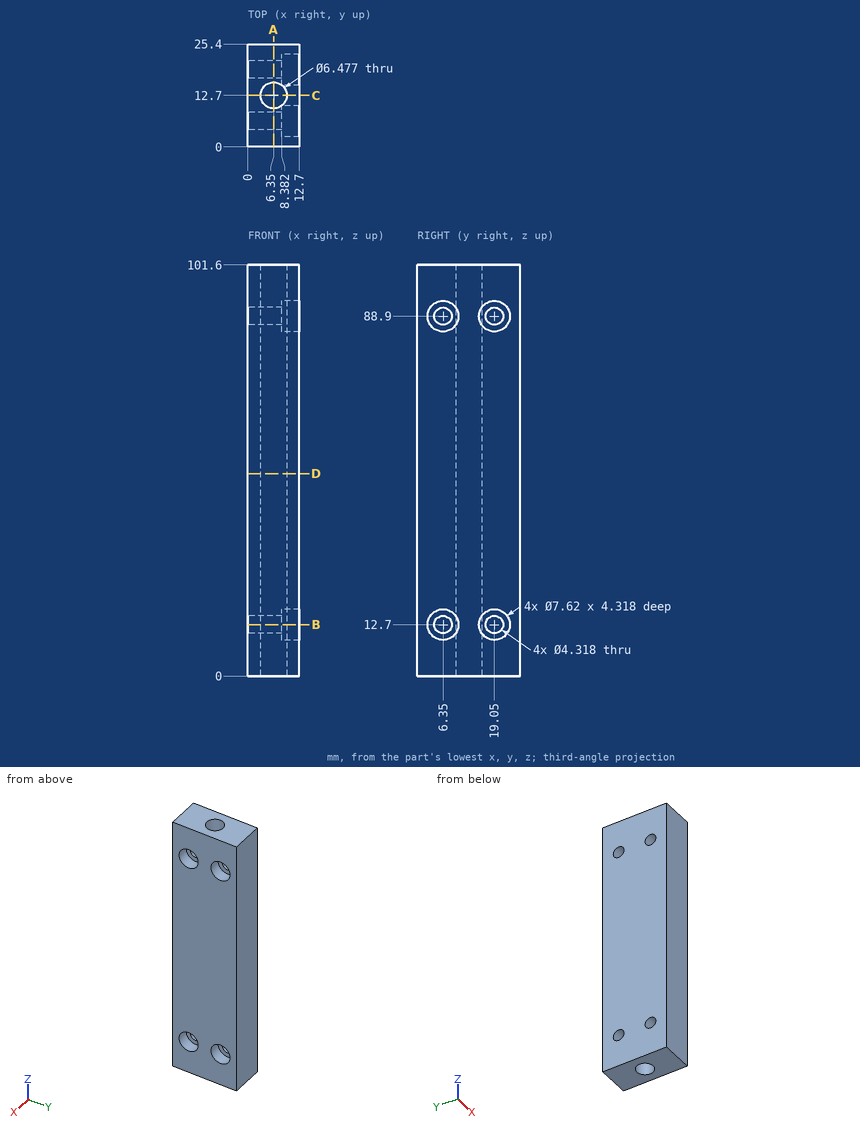
Part print with two shaded views. Sizes in mm from the minimum x, y, z corner. Coordinates: 2 decimals unless noted, no trailing zeros. Order: outer loops, then holes, each group sorted by start corner. A loop starts at its lowest first (then second) coordinate and runs counter-clockwise, first axis right, second up. Notation, with made-up numbers: M 5.5,55 L 38.5,55 A29 ccw 38.5,80 Z; hole C 55.25,20 d3. An arc over 180 degrees is marked long. One line per question, with ' | ' between items. Start each with the question number.
1. Wall check: line 1 along Y through (x, z) = (10.8, 12.7); line 2 along Y through (x, z) = (0.5, 13); line 3 along Z through (x, y) = (2.5, 19.05). Give the ranges that are in metal, low to high. Write a range as [from, to].
2. Cut at A-A (x = 6.35). Write the cut outline in (y, z).
3. Cut at D-D (z = 50). Write the cut outline in (x, y), plus the area to 3 significant figures.
4. Cut at B-B (z = 12.7). Write the cut outline in (x, y), plus the area to 3 significant figures.
5. Flat gauge pin, fed straight in: P1, Ø2.5, axis at y = 7, z = 87, coming from the +X side. Where does the tip first touch, or does it go through?
6. Cut at C-C (y = 12.7). Write the cut outline in (x, z), plus the area to 3 significant figures.
The answers:
1) line 1: y = [0, 2.54], [10.16, 15.24], [22.86, 25.4] | line 2: y = [0, 4.21], [8.49, 16.91], [21.19, 25.4] | line 3: z = [0, 10.54], [14.86, 86.74], [91.06, 101.6]
2) outline: M 0,0 L 9.46,0 L 9.46,101.6 L 0,101.6 Z; M 15.94,0 L 25.4,0 L 25.4,101.6 L 15.94,101.6 Z; hole C 6.35,12.7 d4.32; hole C 6.35,88.9 d4.32; hole C 19.05,12.7 d4.32; hole C 19.05,88.9 d4.32
3) outline: M 0,0 L 12.7,0 L 12.7,25.4 L 0,25.4 Z; hole C 6.35,12.7 d6.48 | area: 290 mm2
4) outline: M 0,0 L 12.7,0 L 12.7,2.54 L 8.38,2.54 L 8.38,4.19 L 0,4.19 Z; M 0,8.51 L 8.38,8.51 L 8.38,10.16 L 12.7,10.16 L 12.7,15.24 L 8.38,15.24 L 8.38,16.89 L 0,16.89 Z; M 0,21.21 L 8.38,21.21 L 8.38,22.86 L 12.7,22.86 L 12.7,25.4 L 0,25.4 Z; hole C 6.35,12.7 d6.48 | area: 151 mm2
5) P1: stops at x = 8.38
6) outline: M 0,0 L 3.11,0 L 3.11,101.6 L 0,101.6 Z; M 9.59,0 L 12.7,0 L 12.7,101.6 L 9.59,101.6 Z | area: 632 mm2
